For this review, take the finished solid that the model builds, in its own axes (mm). A direction names the side the tool comes from. Give positions to 0.01 mm unless a question says otherwise; leave off trailing zeros. Write each loop counter-clockwise with the first axis right and the second up, starting at its lowest first coordinate (ties: lowest second). Pieces come first, ordered by that corner, then holes.
Q1. We need section C-C (z = -0.25). Write out the cut boundary in (x, y) (3 decimals), then the cut area to 3 significant figures.
Q2. We need section B-B (y = 0). Write out the cut boundary in (x, z), then the cut area to 3 significant figures.
Q3. Machinability: for faces 1 (the flat face through (0, 0, 20.1)), 2 (the flat face through (0, -6, 0)), 3 (the cylindrical face through (-0.26, -1.16, 18.43)), which of the approach directions +Z, -Z, +X, -X, +Y, -Y give a long, thin tool a straight path to every point of the face, cutting with its end or side? Answer none if there is none.
Q4. We need section A-A (x = 0). Write out the cut boundary in (y, z), then the cut area to 3 significant figures.
Q5. We need section D-D (x = -5.75). Write out the cut boundary in (y, z), then the cut area to 3 significant figures.
Q6. Insertion check: P1, Ø5, axis at x = -2.5, z = 7.5, coming from the +Y side; P2, Ø8, axis at x = 2, y = 5.5, coming from the +Z side; P3, Ø1.2, axis at x = 1, z = -1, coming from the -Y side; P4, Ø1.5, axis at x = 5.5, z = 9, coming from the +Y side. Each pin has a flat end and moves straight along its axis. Give the tip position at first contact, or say it passes through.
Q7. For line 1 (Y direction, x = -0.25, z = 4.5); line 2 (Z direction, x = 2.25, y = -1.25); line 3 (X direction, y = 3.75, z = 12.5), list the stretches that pass through material, from the lowest coordinate up.
```python
from build123d import *
from build123d.topology import SkipClean

# Parameters (mm, degrees)
ESQUISSE1_R        = 7.5
BOSS_EXTRU_1_DEPTH = 15.05
ESQUISSE3_R        = 6.5
BOSS_EXTRU_2_DEPTH = 0.75
ESQUISSE4_R        = 3
BOSS_EXTRU_3_DEPTH = 1
ESQUISSE5_R        = 1.19
BOSS_EXTRU_4_DEPTH = 3.3
BOSS_EXTRU_7_START = 2.4
BOSS_EXTRU_7_DEPTH = 2.4


with BuildPart() as part:
    # Esquisse1 → Boss.-Extru.1 (new body)
    with BuildSketch(Plane.XY):
        Circle(ESQUISSE1_R)
    extrude(amount=BOSS_EXTRU_1_DEPTH)

    # Esquisse3 → Boss.-Extru.2 (add)
    with BuildSketch(Plane.XY.offset(15.05)):
        Circle(ESQUISSE3_R)
    extrude(amount=BOSS_EXTRU_2_DEPTH)

    # Esquisse4 → Boss.-Extru.3 (add)
    with BuildSketch(Plane.XY.offset(15.8)):
        Circle(ESQUISSE4_R)
    extrude(amount=BOSS_EXTRU_3_DEPTH)

    # Esquisse5 → Boss.-Extru.4 (add)
    with BuildSketch(Plane.XY.offset(16.8)):
        Circle(ESQUISSE5_R)
    extrude(amount=BOSS_EXTRU_4_DEPTH)

    # Esquisse8 → Boss.-Extru.7 (add)
    with SkipClean():  # the faces are left unmerged after this step: merging them gives an invalid solid
        with BuildSketch(Plane(origin=(0, 0, 0), x_dir=(-1, 0, 0), z_dir=(0, 0, -1)).offset(BOSS_EXTRU_7_START)):
            with BuildLine():
                Line((-4.754997371, -5.8), (4.754997371, -5.8))
                ThreePointArc((4.754997371, -5.8), (0, 7.5), (-4.754997371, -5.8))
            make_face()
        extrude(amount=-BOSS_EXTRU_7_DEPTH)


solid = part.part
```
Computed:
1. outline: (-4.755, -5.8) - (4.755, -5.8) arc R7.5 ccw (long way) to start
1. area: 166 mm2
2. outline: (-7.5, -2.4) - (7.5, -2.4) - (7.5, 15.05) - (6.5, 15.05) - (6.5, 15.8) - (3, 15.8) - (3, 16.8) - (1.19, 16.8) - (1.19, 20.1) - (-1.19, 20.1) - (-1.19, 16.8) - (-3, 16.8) - (-3, 15.8) - (-6.5, 15.8) - (-6.5, 15.05) - (-7.5, 15.05) - close
2. area: 285 mm2
3. face 1: +Z, +X, -X, +Y, -Y
3. face 2: -Z, +X, -X, -Y
3. face 3: +Z
4. outline: (-7.5, 0) - (-5.8, 0) - (-5.8, -2.4) - (7.5, -2.4) - (7.5, 15.05) - (6.5, 15.05) - (6.5, 15.8) - (3, 15.8) - (3, 16.8) - (1.19, 16.8) - (1.19, 20.1) - (-1.19, 20.1) - (-1.19, 16.8) - (-3, 16.8) - (-3, 15.8) - (-6.5, 15.8) - (-6.5, 15.05) - (-7.5, 15.05) - close
4. area: 281 mm2
5. outline: (-4.82, -2.4) - (4.82, -2.4) - (4.82, 15.05) - (3.03, 15.05) - (3.03, 15.8) - (-3.03, 15.8) - (-3.03, 15.05) - (-4.82, 15.05) - close
5. area: 173 mm2
6. P1: stops at y = 7.5
6. P2: stops at z = 16.8
6. P3: stops at y = -5.8
6. P4: stops at y = 5.8
7. line 1: y = -7.5 to 7.5
7. line 2: z = -2.4 to 16.8
7. line 3: x = -6.5 to 6.5
